Autodesk Inventor part; units mm, degrees
ref_plane "Work Plane1" through (-2.667, -3.175, 0.508) normal (-1, 0, 0) x (0, 0, -1)
ref_plane "YZ Plane" through (0, 0, 0) normal (1, 0, 0) x (0, 1, 0)
ref_plane "XZ Plane" through (0, 0, 0) normal (0, 1, 0) x (-1, 0, 0)
sketch "Sketch1" plane through (0, 0, 0) normal (0, 0, 1) x (1, 0, 0)
  line L0 (-3.175, 3.175) -> (3.175, 3.175)
  line L1 (3.175, 3.175) -> (3.175, -3.175)
  line L2 (3.175, -3.175) -> (-3.175, -3.175)
  line L3 (-3.175, -3.175) -> (-3.175, 3.175)
  line L4 (0, 0) -> (0, 0.9618)
  line L5 (0, 0) -> (0.9618, 0)
  dimension "d0" = 6.35
extrude "Extrusion1" add sketch "Sketch1" along normal blind 3.175
sketch "Sketch2" plane through (0, 0, 3.175) normal (0, 0, 1) x (1, 0, 0)
  circle A0 centre (0, 0) radius 1.651
  dimension "d3" = 3.302
extrude "Extrusion2" add sketch "Sketch2" along normal blind 4.1656
sketch "Sketch3" plane through (0, 0, 3.175) normal (0, 0, 1) x (1, 0, 0)
  circle A0 centre (0, 0) radius 1.651
  circle A1 centre (0, 0) radius 3.175
  line L0 (0, 0) -> (3.175, 3.175)
  circle A2 centre (2.2451, 2.2451) radius 0.3175
  dimension "d6" = 0.635
extrude "Extrusion3" add sketch "Sketch3" along normal blind 0.508 contours A2 A1 L0 | L0 A1 A2 | L0 A2 A1 | A1 A2 L0
pattern_circular "Circular Pattern1" count 4 over 360 about axis through (0, 0, 3.175) along (0, 0, 1) of "Extrusion3"
sketch "Sketch4" plane through (0, 0, 3.175) normal (0, 0, 1) x (1, 0, 0)
  circle A0 centre (2.2451, -2.2451) radius 0.3175
  circle A1 centre (-2.2451, -2.2451) radius 0.3175
  circle A2 centre (-2.2451, 2.2451) radius 0.3175
  circle A3 centre (2.2451, 2.2451) radius 0.3175
  circle A4 centre (0, 0) radius 1.651
  line L0 (3.175, 3.175) -> (3.175, -3.175)
  line L1 (-3.175, 3.175) -> (3.175, 3.175)
  line L2 (-3.175, -3.175) -> (-3.175, 3.175)
  line L3 (3.175, -3.175) -> (-3.175, -3.175)
  line L4 (3.1021, 3.1021) -> (3.1021, -3.1021)
  line L5 (3.1021, -3.1021) -> (-3.1021, -3.1021)
  line L6 (-3.1021, -3.1021) -> (-3.1021, 3.1021)
  line L7 (-3.1021, 3.1021) -> (3.1021, 3.1021)
extrude "Extrusion4" add sketch "Sketch4" along normal blind 0.381 contours L4 L5 L6 L7
sketch "Sketch5" plane through (-3.175, -3.175, 0) normal (0, -1, 0) x (1, 0, 0)
  line L0 (0, 0) -> (0, 3.175)
  line L1 (6.35, 0) -> (0, 0)
  line L2 (0.127, 0.508) -> (0.508, 0.508)
  line L3 (0.508, 0.508) -> (0.508, 0.254)
  line L4 (0.508, 0.254) -> (0.127, 0.254)
  line L5 (0.127, 0.254) -> (0.127, 0.508)
  dimension "d14" = 0.381
  dimension "d15" = 0.254
  dimension "d16" = 0.127
  dimension "d17" = 0.254
ref_plane "Work Plane1" through (-2.667, -3.175, 0.508) normal (-1, 0, 0) x (0, 0, -1)
sketch "Sketch6" plane through (-2.667, -3.175, 0.508) normal (-1, 0, 0) x (0, 0, -1)
  line L0 (0, -0.1801) -> (0, 0.0739)
  line L1 (0.254, 0.3279) -> (1.016, 0.3279)
  arc A0 (0.254, 0.3279) -> (0, 0.0739) centre (0.254, 0.0739) ccw
  point P0 (0, 0.3279)
  dimension "d19" = 0.508
  dimension "d20" = 1.016
  dimension "d21" = 0.254
sweep "Sweep1" add profiles "Sketch5" path "Sketch6"
mirror "Mirror1" about plane through (0, 0, 0) normal (1, 0, 0) of "Sweep1"
mirror "Mirror2" about plane through (0, 0, 0) normal (0, 1, 0) of "Sweep1", "Mirror1"
properties part number "cRIO-FRC Switch" material "ABS Plastic"
The model under review builds one solid part; all positions refer to its coordinate system, in mm. A direction names the side the tool comes from. Round coordinates to 2 decimals unless told otherwise and drop trailing zeros. Loops run counter-clockwise (first coordinate to the right, second up) from the corner with the lowest first, then second, coordinate; pieces in that order, holes last. Notation, with made-up numbers: (-7.75, -11) -> (3.25, -11) arc R9 cw to (3.25, -6) -> close; hole circle Ø7 at (88.5, 47.5). An arc over 180 degrees is marked (long way). Answer in a Markdown table with one row per item.
1) For pin 1 Ø1 at (x, y) = (2, 1) entering from +Z; pin 2 Ø1.5 at (x, z) = (-1.5, 6.5) entering from +Y; pin 3 Ø0.7 at (x, y) = (-2, 2.5) entering from +Z, all flat-tipped, find the tip position at first contact; note any pin that passes through.
Taken from the geometry:
| item | result |
|---|---|
| pin 1 | stops at z = 3.56 |
| pin 2 | stops at y = 1.47 |
| pin 3 | stops at z = 3.68 |
2) Wall thickness on line 1 along Z through (x, y) = (0.5, -2.75); line 2 along Y through (x, z) = (0, 1.5) (3 decimals); line 3 along X through (y, z) = (2.25, 3.5): over which ranges is each line inside the solid? List them lowest first.
Taken from the geometry:
| item | result |
|---|---|
| line 1 | z = 0 to 3.56 |
| line 2 | y = -3.175 to 3.175 |
| line 3 | x = -3.1 to 3.1 |
3) Tool access review of faces 1 (the flat face through (0, 0, 7.341)), 2 (the flat face through (0, 0, 0)): name each direction out of +Z, -Z, +X, -X, +Y, -Y from which nothing blocks a thin tool from reaching the whole face with its end or side.
Taken from the geometry:
| item | result |
|---|---|
| face 1 | +Z, +X, -X, +Y, -Y |
| face 2 | -Z, +X, -X |
4) Consider section A-A, the plane y = 0. Write out the cut boundary in (x, z) (3 decimals), plus the area to 3 significant figures.
Taken from the geometry:
| item | result |
|---|---|
| outline | (-3.175, 0) -> (3.175, 0) -> (3.175, 3.175) -> (3.102, 3.175) -> (3.102, 3.556) -> (1.651, 3.556) -> (1.651, 7.341) -> (-1.651, 7.341) -> (-1.651, 3.556) -> (-3.102, 3.556) -> (-3.102, 3.175) -> (-3.175, 3.175) -> close |
| area | 35.0 mm² |
5) Consider section C-C, the plane z = 6. Write out the cut boundary in (x, y), plus the area to 3 significant figures.
Taken from the geometry:
| item | result |
|---|---|
| outline | circle Ø3.3 at (0, 0) |
| area | 8.56 mm² |
6) Consider section D-D, the plane z = 0.75. Write out the cut boundary in (x, y) (3 decimals).
Taken from the geometry:
| item | result |
|---|---|
| outline | (-3.175, -3.175) -> (3.175, -3.175) -> (3.175, 3.175) -> (-3.175, 3.175) -> close |
7) Draft analysis for pull direction X (two halves, no side actions). For faces 3 (the flat face through (3.175, 0, 2)), 4 (the flat face through (-1.4, -1.3, 3.556)), 5 (the cylindrical face through (1.525, 0.632, 5.422)), state which applies: pulls with the +X half, pulls with the -X half, needs draft (parallel to the pull), parting line crosses it, or undercut.
Taken from the geometry:
| item | result |
|---|---|
| face 3 | pulls with the +X half |
| face 4 | undercut |
| face 5 | parting line crosses it |
